Could you check a few things on this model? Use its own coordinates, in mm. Give positions to 0.01 mm unless a question says otherwise; leave off trailing zeros. Order: outer loops, then holes, each group sorted by start corner. A loop starts at its lowest first (then second) coordinate and runs counter-clockwise, first axis right, second up. Notation, with made-up numbers: M 37.25,55 L 85.25,55 A34 cw 85.25,87 Z; hole C -33,-20 d10. An arc over 180 degrees is marked long. Use a Markdown table: item, result. Add a question column.
Item 1: Suppose I cut it at A-A on z = 604. Write out the boundary of the cut face in (x, y), plus the area to 3 significant figures.
Item 2: Suppose I cut it at B-B on y = -133. Write out the boundary of the cut face in (x, z), plus the area to 3 significant figures.
Item 3: I'm going to push flat-ended pins straight in: pin 1 Ø0.5 at (x, y) = (-780.5, 400.5) entering from +Z; pin 2 Ø24 at (x, z) = (135.5, 718.5) entering from +Y; pin 3 Ø9 at (y, z) = (-161.5, 715.5) entering from -X. Where does each tip first touch, or does it pass through?
Item 4: If I drill on L1, parallel to Z at x = 552.5, y = 349, over which ranges is the centre line in solid material (lowest first)? Write a range as from..to.
Item 5: Suppose I cut it at C-C on x = 388.5. Write out the boundary of the cut face in (y, z), plus the area to 3 significant figures.
from build123d import *

# Parameters (mm, degrees)
CYLINDER002_R     = 20
CYLINDER002_DEPTH = 700
CYLINDER001_R     = 20
CYLINDER001_DEPTH = 700
CYLINDER_R        = 20
CYLINDER_DEPTH    = 700
BOX_W             = 1600
BOX_H             = 800
BOX_DEPTH         = 30
CYLINDER003_R     = 20
CYLINDER003_DEPTH = 700


with BuildPart() as cylinder002:
    # Cylinder002 → Cylinder002 (new body)
    with BuildSketch(Plane(origin=(-780, 381, 0), x_dir=(1, 0, 0), z_dir=(0, 0, 1))):
        Circle(CYLINDER002_R)
    extrude(amount=CYLINDER002_DEPTH)


with BuildPart() as cylinder001:
    # Cylinder001 → Cylinder001 (new body)
    with BuildSketch(Plane(origin=(780, -380, 0), x_dir=(1, 0, 0), z_dir=(0, 0, 1))):
        Circle(CYLINDER001_R)
    extrude(amount=CYLINDER001_DEPTH)


with BuildPart() as cylinder:
    # Cylinder → Cylinder (new body)
    with BuildSketch(Plane(origin=(780, 380, 0), x_dir=(1, 0, 0), z_dir=(0, 0, 1))):
        Circle(CYLINDER_R)
    extrude(amount=CYLINDER_DEPTH)


with BuildPart() as cube:
    # Box → Box (new body)
    with BuildSketch(Plane(origin=(-800, -400, 700), x_dir=(1, 0, 0), z_dir=(0, 0, 1))):
        with Locations((800, 400)):
            Rectangle(BOX_W, BOX_H)
    extrude(amount=BOX_DEPTH)


with BuildPart() as fusion:
    # Cylinder003 → Cylinder003 (new body)
    with BuildSketch(Plane(origin=(-781, -380, 0), x_dir=(1, 0, 0), z_dir=(0, 0, 1))):
        Circle(CYLINDER003_R)
    extrude(amount=CYLINDER003_DEPTH)

    # Fusion: union Cylinder002, Cylinder001, Cylinder, Cube
    add(cylinder002.part)
    add(cylinder001.part)
    add(cylinder.part)
    add(cube.part)


solid = fusion.part
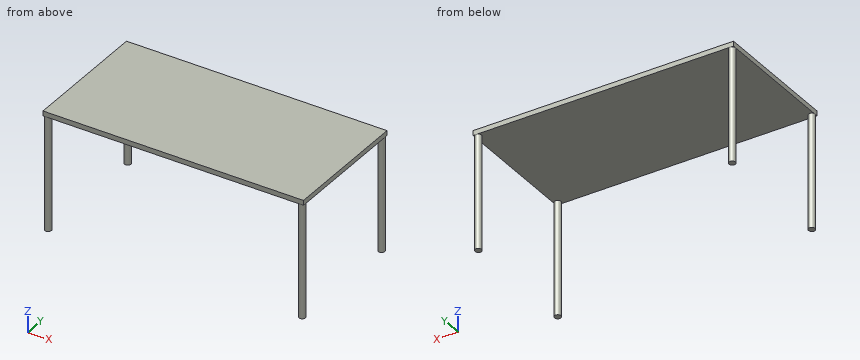
Findings below:
| question | item | result |
|---|---|---|
| 1 | outline | C -781,-380 d40; C -780,381 d40; C 780,-380 d40; C 780,380 d40 |
| 1 | area | 5,030 mm^2 |
| 2 | outline | M -800,700 L 800,700 L 800,730 L -800,730 Z |
| 2 | area | 48,000 mm^2 |
| 3 | pin 1 | stops at z = 700 |
| 3 | pin 2 | stops at y = 400 |
| 3 | pin 3 | stops at x = -800 |
| 4 | L1 | z = 700..730 |
| 5 | outline | M -400,700 L 400,700 L 400,730 L -400,730 Z |
| 5 | area | 24,000 mm^2 |
